Verification items for the finished model (mm, model axes). A direction names the side the tool comes from. Coordinates: 2 decimals unless noted, no trailing zeros. Write each loop counter-clockwise with the first axis right and the second up, starting at its lowest first coordinate (ties: lowest second). Pieces come first, ordered by that corner, then holes. Notation, with made-up numbers: (39.5, -7.5) -> (81.5, -7.5) arc R33 cw to (81.5, 21.5) -> close; hole circle Ø4 at (6.5, 88). An arc over 180 degrees is marked (long way). Use CSV: the item, a comma, the result in double quotes.
```python
from build123d import *

# Parameters (mm, degrees)
SKETCH2_R           = 9.525
SKETCH2_W           = 60.325
SKETCH2_H           = 15.875
BOSS_EXTRUDE1_DEPTH = 12.7
SKETCH2_4_W         = 60.325
SKETCH2_4_H         = 15.875
BOSS_EXTRUDE2_DEPTH = 122.2375
BOSS_EXTRUDE4_START = 122.2375
SKETCH2_7_W         = 60.325
SKETCH2_7_H         = 15.875
BOSS_EXTRUDE4_DEPTH = 23.8125
BOSS_EXTRUDE5_START = 133.35
SKETCH2_9_R         = 19.05
SKETCH2_9_R_2       = 9.525
BOSS_EXTRUDE5_DEPTH = 12.7
FILLET1_R           = 6.35
SKETCH3_R           = 6.746875
CUT_EXTRUDE1_DEPTH  = 75.6125


with BuildPart() as part:
    # Sketch2 → Boss-Extrude1 (new body)
    with BuildSketch(Plane(origin=(0, 0, 0), x_dir=(0, 0, -1), z_dir=(1, 0, 0))):
        with BuildLine():
            Line((60.325, 15.875), (60.325, 47.625))
            ThreePointArc((60.325, 47.625), (30.1625, 77.7875), (0, 47.625))
            Line((0, 47.625), (0, 15.875))
            Line((0, 15.875), (60.325, 15.875))
        make_face()
        with Locations((30.1625, 47.625)):
            Circle(SKETCH2_R, mode=Mode.SUBTRACT)
        with Locations((30.1625, 7.9375)):
            Rectangle(SKETCH2_W, SKETCH2_H)
    extrude(amount=BOSS_EXTRUDE1_DEPTH)

    # Sketch2_4 → Boss-Extrude2 (add)
    with BuildSketch(Plane(origin=(0, 0, 0), x_dir=(0, 0, -1), z_dir=(1, 0, 0))):
        with Locations((30.1625, 7.9375)):
            Rectangle(SKETCH2_4_W, SKETCH2_4_H)
    extrude(amount=BOSS_EXTRUDE2_DEPTH)

    # Sketch2_7 → Boss-Extrude4 (add)
    with BuildSketch(Plane(origin=(0, 0, 0), x_dir=(0, 0, -1), z_dir=(1, 0, 0)).offset(BOSS_EXTRUDE4_START)):
        with BuildLine():
            Line((60.325, 0), (0, 0))
            Line((0, 0), (0, -3.175))
            ThreePointArc((0, -3.175), (2.430039796, -3.658364969), (4.490128061, -5.034871939))
            Line((4.490128061, -5.034871939), (30.540891087, -4.907791916))
            ThreePointArc((30.540891087, -4.907791916), (33.205851981, -4.762821099), (35.872100396, -4.881785376))
            Line((35.872100396, -4.881785376), (60.325, -4.7625))
            Line((60.325, -4.7625), (60.325, 0))
        make_face()
        with Locations((30.1625, 7.9375)):
            Rectangle(SKETCH2_7_W, SKETCH2_7_H)
        with BuildLine():
            ThreePointArc((35.872100396, -4.881785376), (33.205851981, -4.762821099), (30.540891087, -4.907791916))
            Line((30.540891087, -4.907791916), (35.872100396, -4.881785376))
        make_face()
    extrude(amount=BOSS_EXTRUDE4_DEPTH)

    # Sketch2_9 → Boss-Extrude5 (add)
    with BuildSketch(Plane(origin=(0, 0, 0), x_dir=(0, 0, -1), z_dir=(1, 0, 0)).offset(BOSS_EXTRUDE5_START)):
        with BuildLine():
            Line((30.540891087, -4.907791916), (4.490128061, -5.034871939))
            ThreePointArc((4.490128061, -5.034871939), (5.866635031, -7.094960204), (6.35, -9.525))
            Line((6.35, -9.525), (6.35, -31.75))
            ThreePointArc((6.35, -31.75), (13.290073241, -13.682741309), (30.540891087, -4.907791916))
        make_face()
        with BuildLine():
            Line((35.872100396, -4.881785376), (30.540891087, -4.907791916))
            ThreePointArc((30.540891087, -4.907791916), (13.290073241, -13.682741309), (6.35, -31.75))
            ThreePointArc((6.35, -31.75), (33.3375, -58.7375), (60.325, -31.75))
            ThreePointArc((60.325, -31.75), (53.296554141, -13.585162703), (35.872100396, -4.881785376))
        make_face()
        with Locations((33.3375, -31.75)):
            Circle(SKETCH2_9_R, mode=Mode.SUBTRACT)
        with Locations((33.3375, -31.75)):
            Circle(SKETCH2_9_R)
        with Locations((33.3375, -31.75)):
            Circle(SKETCH2_9_R_2, mode=Mode.SUBTRACT)
        with BuildLine():
            Line((60.325, -31.75), (60.325, -4.7625))
            Line((60.325, -4.7625), (35.872100396, -4.881785376))
            ThreePointArc((35.872100396, -4.881785376), (53.296554141, -13.585162703), (60.325, -31.75))
        make_face()
    extrude(amount=BOSS_EXTRUDE5_DEPTH)

    # Fillet1
    fillet1_edges = [part.edges().sort_by_distance(p)[0] for p in [
        (12.7, 15.875, -30.1625),
        (146.05, 15.875, -30.1625),
    ]]
    fillet(fillet1_edges, radius=FILLET1_R)

    # Sketch3 → Cut-Extrude1 (cut, through all)
    with BuildSketch(Plane(origin=(0, 15.875, 0), x_dir=(1, 0, 0), z_dir=(0, 1, 0))):
        with Locations((53.975, 30.1625)):
            Circle(SKETCH3_R)
        with Locations((123.825, 30.1625)):
            Circle(SKETCH3_R)
    extrude(amount=-CUT_EXTRUDE1_DEPTH, mode=Mode.SUBTRACT)


solid = part.part
```
1) Mould release check, pull along Y, two halves, no side actions. Record for faces 6 (the flat face through (12.7, 38, -36)), 7 (the cylindrical face through (139.61, -40.2, -37.73)), 8 (the cylindrical face through (6.26, 77.78, -30.83)): released by +Y, released by -Y, zero draft, split by the parting line, or undercut.
Return value:
face 6,"zero draft"
face 7,"undercut"
face 8,"released by +Y"
2) Set-up check for faces 1 (the flat face through (79, 15.875, -30)), 2 (the cylindrical face through (139.61, -58.73, -32.74)), 3 (the flat face through (122.238, -2, -48)), 4 (the flat face through (140, -20, -6.35)), 5 (the flat face through (73, 8, -60.325)): record each of +Z, -Z, +X, -X, +Y, -Y from which the full face is reachable in a straight line by a thin tool's end or side.
Return value:
face 1,"+Z, -Z, +X, +Y"
face 2,"+X, -X, -Y"
face 3,"+Z, -Z, -X, -Y"
face 4,"+Z, +X, -X, -Y"
face 5,"-Z, +X, -X, +Y, -Y"
3) Cross-section at C-C (x = 42.5). Record the boundary of the cut face in (y, z) (3 decimals).
Return value:
outline,"(0, -60.325) -> (15.875, -60.325) -> (15.875, 0) -> (0, 0) -> close"
4) Gauge pin test, flat ends, axial feed: pin 1 (18 mm diameter, centred on x = 79, z = -22, fed in from -Y); pin 2 (1 mm diameter, centred on y = -24.5, z = -24, fed in from -X); pin 3 (2 mm diameter, centred on y = 22.5, z = -13.5, fed in from +X); pin 4 (1.5 mm diameter, centred on y = 37.5, z = -11, fed in from -X). Record the tip position at first contact, or that the pin passes through.
Return value:
pin 1,"y = 0"
pin 2,"x = 133.35"
pin 3,"x = 12.74"
pin 4,"x = 0"
5) Scan lines: L1, parallel to X at y = 39, z = -41.5; L2, parallel to Y at x = 121.5, z = -44.5 (3 decimals); L3, parallel to X at y = -18, z = -56.5. Record each from-to range of solid material in increasing order.
Return value:
L1,"0 to 12.7"
L2,"0 to 15.875"
L3,"133.35 to 146.05"
6) Cross-section at B-B (y = 13). Record the boundary of the cut face in (x, z) (1 decimal), plus the area to 3 significant figures.
Return value:
outline,"(0, -60.3) -> (145, -60.3) -> (145, 0) -> (0, 0) -> close; hole circle Ø13.5 at (54, -30.2); hole circle Ø13.5 at (123.8, -30.2)"
area,"8,460 mm2"
7) Cross-section at D-D (y = 68). Record the boundary of the cut face in (x, z).
Return value:
outline,"(0, -52.4) -> (12.7, -52.4) -> (12.7, -7.92) -> (0, -7.92) -> close"
